Check sheet for the drawn part. Datum: minimum x, y, z corner. Units: mm. Give positions to 0.01 mm unless a question says otherwise; leave off trailing zeros. Order: outer loops, then holes, each group sorted by start corner. A loop starts at its lowest first (then second) coordinate and runs counter-clockwise, first axis right, second up.
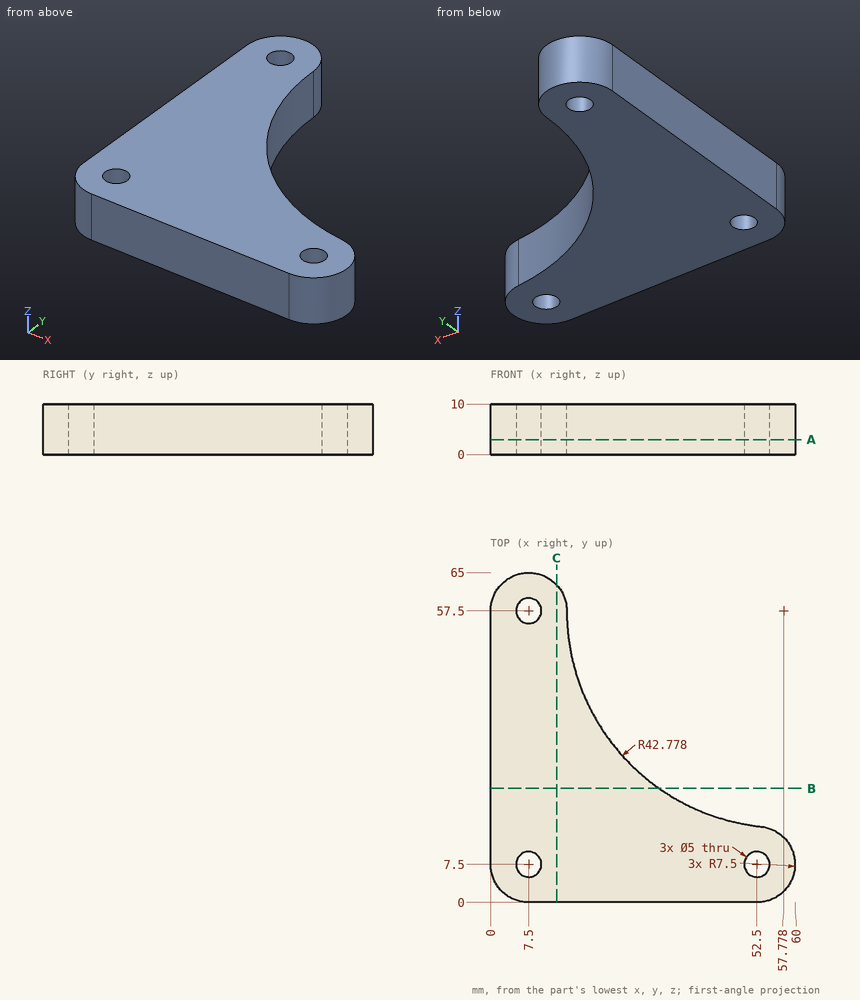
(1) Section check B-B, the plane y = 22.5. Enter the section's corners in (x, z), then the cut area to 3 significant figures.
Solved:
outline: (0, 0) - (33.18, 0) - (33.18, 10) - (0, 10) - close
area: 332 mm2
(2) Scan lines: line 1 (Y direction, x = 7.5, z = 8); line 2 (X direction, y = 9.5, z = 8.5); line 3 (X direction, y = 58, z = 3.75). Record each from-to range of solid material in increasing order.
Solved:
line 1: y = 0 to 5, 10 to 55, 60 to 65
line 2: x = 0 to 6, 9 to 51, 54 to 59.73
line 3: x = 0.02 to 5.05, 9.95 to 14.98
(3) Section check C-C, the plane x = 13. Enter the section's corners in (y, z).
Solved:
outline: (0, 0) - (62.6, 0) - (62.6, 10) - (0, 10) - close
(4) Section check A-A, the plane z = 3. Enter the section's corners in (x, y).
Solved:
outline: (0, 7.5) arc R7.5 ccw to (7.5, 0) - (52.5, 0) arc R7.5 ccw to (53.29, 14.96) arc R42.78 cw to (15, 57.5) arc R7.5 ccw to (0, 57.5) - close; hole circle Ø5 at (7.5, 7.5); hole circle Ø5 at (7.5, 57.5); hole circle Ø5 at (52.5, 7.5)
(5) Go/stop test with flat-tipped pins: pin 1 (5 mm diameter, centred on x = 24.5, z = 1.5, fed in from +Y); pin 2 (1.5 mm diameter, centred on x = 17, y = 51.5, fed in from +Z); pin 3 (4 mm diameter, centred on y = 49.5, z = 6, fed in from +X) (1 decimal). Record where each tip stops, or that it passes through.
Solved:
pin 1: stops at y = 34.05
pin 2: passes through
pin 3: stops at x = 16.2
